from build123d import *

# Parameters (mm, degrees)
BOSS_EXTRUDE1_DEPTH = 6
SKETCH6_W           = 87
SKETCH6_H           = 6.5
BOSS_EXTRUDE2_DEPTH = 2
SKETCH7_W           = 97
SKETCH7_H           = 16.106562898
SKETCH7_W_2         = 87
SKETCH7_H_2         = 6.5
BOSS_EXTRUDE3_DEPTH = 5
SKETCH8_R           = 2
CUT_EXTRUDE1_DEPTH  = 138.309868546
SKETCH10_W          = 4
SKETCH10_H          = 6.5
BOSS_EXTRUDE4_DEPTH = 9
SKETCH11_R          = 3
CUT_EXTRUDE2_DEPTH  = 21
FILLET1_R           = 1


with BuildPart() as part:
    # Sketch1 → Boss-Extrude1 (new body)
    with BuildSketch(Plane(origin=(0, 0, 0), x_dir=(1, 0, 0), z_dir=(0, 1, 0))):
        Polygon((0, 7), (0, 0), (7, 0), (90, 0), (97, 0), (97, 7), (97, 90), (97, 97), (90, 97), (7, 97), (0, 97), (0, 90), align=None)
        Polygon((7, 7), (5, 7), (5, 11.893437102), (92, 11.893437102), (92, 7), (90, 7), (90, 5), (7, 5), align=None, mode=Mode.SUBTRACT)
        Polygon((5, 23), (92, 23), (92, 16.5), (5, 16.5), (5, 16.893437102), align=None, mode=Mode.SUBTRACT)
        Polygon((7, 92), (90, 92), (90, 90), (92, 90), (92, 28), (5, 28), (5, 90), (7, 90), align=None, mode=Mode.SUBTRACT)
    extrude(amount=BOSS_EXTRUDE1_DEPTH)

    # Sketch6 → Boss-Extrude2 (add)
    with BuildSketch(Plane.XZ):
        with Locations((48.5, -19.75)):
            Rectangle(SKETCH6_W, SKETCH6_H)
    extrude(amount=-BOSS_EXTRUDE2_DEPTH)

    # Sketch7 → Boss-Extrude3 (add)
    with BuildSketch(Plane(origin=(0, 6, 0), x_dir=(1, 0, 0), z_dir=(0, 1, 0))):
        with Locations((48.5, 19.946718551)):
            Rectangle(SKETCH7_W, SKETCH7_H)
        with Locations((48.5, 19.75)):
            Rectangle(SKETCH7_W_2, SKETCH7_H_2, mode=Mode.SUBTRACT)
    extrude(amount=BOSS_EXTRUDE3_DEPTH)

    # Sketch8 → Cut-Extrude1 (cut, through all)
    with BuildSketch(Plane(origin=(0, 6, 0), x_dir=(1, 0, 0), z_dir=(0, 1, 0))):
        with Locations(Location((93.5, 93.5, 0), (0, 0, 270))):
            Circle(SKETCH8_R)
        with Locations(Location((3.5, 3.5, 0), (0, 0, 270))):
            Circle(SKETCH8_R)
        with Locations(Location((3.5, 93.5, 0), (0, 0, 270))):
            Circle(SKETCH8_R)
        with Locations(Location((93.5, 3.5, 0), (0, 0, 270))):
            Circle(SKETCH8_R)
    extrude(amount=-CUT_EXTRUDE1_DEPTH, mode=Mode.SUBTRACT)

    # Sketch10 → Boss-Extrude4 (add)
    with BuildSketch(Plane(origin=(0, 2, 0), x_dir=(1, 0, 0), z_dir=(0, 1, 0))):
        with Locations((90, 19.75)):
            Rectangle(SKETCH10_W, SKETCH10_H)
        with Locations((7, 19.75)):
            Rectangle(SKETCH10_W, SKETCH10_H)
    extrude(amount=BOSS_EXTRUDE4_DEPTH)

    # Sketch11 → Cut-Extrude2 (cut)
    with BuildSketch(Plane(origin=(0, 11, 0), x_dir=(1, 0, 0), z_dir=(0, 1, 0))):
        with Locations(Location((92.5, 19.946718551, 0), (0, 0, 270))):
            Circle(SKETCH11_R)
        with Locations(Location((4.5, 19.946718551, 0), (0, 0, 270))):
            Circle(SKETCH11_R)
    extrude(amount=-CUT_EXTRUDE2_DEPTH, mode=Mode.SUBTRACT)

    # Fillet1
    fillet1_edges = [part.edges().sort_by_distance(p)[0] for p in [
        (88, 6.5, -23),
        (88, 6.5, -16.5),
        (9, 6.5, -16.5),
        (9, 6.5, -23),
    ]]
    fillet(fillet1_edges, radius=FILLET1_R)


solid = part.part
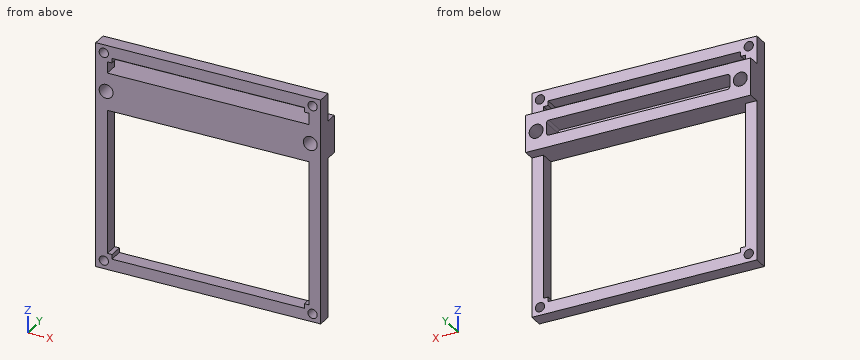
Could you check a few things on this model? Use its own coordinates, in mm. Give positions to 0.01 mm unless a question says otherwise; leave off trailing zeros. Order: outer loops, then holes, each group sorted by start corner. A loop starts at its lowest first (then second) coordinate and runs counter-clockwise, first axis right, second up. Notation, with made-up numbers: (45.5, -16) - (69.5, -16) arc R23 cw to (69.5, -5) - close; hole circle Ø11 at (-11, -13). An arc over 180 degrees is marked (long way). Return JSON: item names as keys, results as strings. Group by question number.
Q1. Please list where these lines run through material, in increasing order: line 1 along Z through (x, y) = (56, 1.5); line 2 along X through (y, z) = (2.8, -3.5); line 3 along Z through (x, y) = (30.5, 4.5). Write a range as [from, to].
Q2. Suppose I cut it at B-B, the plane y = 8.5. Please give me the cut outline in (x, z), and give its area (3 significant figures).
Q3. Will these pins go through, and if not, where does the flat tip stop? pin 1 Ø5 at (x, z) = (81, -20) entering from +Y; pin 2 Ø3.5 at (x, z) = (49, -6.5) entering from +Y.
Q4. Suppose I cut it at A-A, the plane z = -86. Please give me the cut outline in (x, y).
Q5. Suppose I cut it at C-C, the plane x = 74. Please give me the cut outline in (y, z), and give its area (3 significant figures).
Q6. Suppose I cut it at D-D, the plane y = 3.5. State how many separate pieces and enclosed holes the cut face has, and give its area (3 significant figures).
Resolved:
{
 "1": {"line 1": "z = [-97, -92], [-28, -11.89], [-5, 0]", "line 2": "x = [0, 1.5], [5.5, 91.5], [95.5, 97]", "line 3": "z = [-97, -92], [-28, -23], [-16.5, -11.89], [-5, 0]"},
 "2": {"outline": "(0, -28) - (97, -28) - (97, -11.89) - (0, -11.89) - close; hole circle Ø6 at (4.5, -19.95); hole (9, -22) arc R1 ccw to (10, -23) - (87, -23) arc R1 ccw to (88, -22) - (88, -17.5) arc R1 ccw to (87, -16.5) - (10, -16.5) arc R1 ccw to (9, -17.5) - close; hole circle Ø6 at (92.5, -19.95)", "area": "993 mm2"},
 "3": {"pin 1": "stops at y = 2", "pin 2": "stops at y = 6"},
 "4": {"outline": "(0, 0) - (5, 0) - (5, 6) - (0, 6) - close; (92, 0) - (97, 0) - (97, 6) - (92, 6) - close"},
 "5": {"outline": "(0, -97) - (6, -97) - (6, -92) - (0, -92) - close; (0, -28) - (11, -28) - (11, -23) - (2, -23) - (2, -16.5) - (11, -16.5) - (11, -11.89) - (0, -11.89) - close; (0, -5) - (6, -5) - (6, 0) - (0, 0) - close", "area": "179 mm2"},
 "6": {"separate pieces": "1", "enclosed holes": "9", "area": "2,640 mm2"}
}
